Could you check a few things on this model? Use its own coordinates, in mm. Face numbers are marked on the shaded views. A direction names the side the tool comes from. Give positions to 0.01 mm unless a question says otherwise; leave off trailing zeros. Order: outer loops, then holes, each group sorted by start corner. A loop starts at its lowest first (then second) coordinate and runs counter-clockwise, first axis right, second up.
(1) If we mould it in two halves opening along Z, with no side actions, what happens to the marked faces 1, 2 and 3? For each: released by +Z, released by -Z, zero draft, split by the parting line, or undercut.
(2) Imagine slicing it at B-B, the plane z = 4.75. Write out the boundary of the cut face in (x, y).
(3) Imagine slicing it at C-C, the plane x = 11. Write out the boundary of the cut face in (y, z).
(4) If I drill on probe 1 along X at (y, z) = (3, -1); probe 2 along Z at (x, y) = (-15, 3); probe 3 along Z at (x, y) = (19, 5.75), over which ranges is the centre line in solid material (lowest first)?
(5) Imagine slicing it at A-A, the plane y = 4.5. Write out the boundary of the cut face in (x, z), then the cut area to 3 significant figures.
(6) Imagine slicing it at D-D, the plane z = 2. Write out the boundary of the cut face in (x, y), then the cut area to 3 significant figures.
(7) Will these pins go through, and if not, where does the flat tip stop? pin 1 (1 mm diameter, centred on y = 4.5, z = -7, fed in from +X); pin 2 (11 mm diameter, centred on x = 10.5, z = -1.5, fed in from +Y); pin 3 (1.6 mm diameter, centred on y = 4.5, z = -8, fed in from -X).
(8) On a 3-axis mill with a long thin cutter (end or side, diameter ignored), from which of +Z, -Z, +X, -X, +Y, -Y can I reach the whole of each face in a straight line? I mean the marked faces 4 and 5. Say none if no direction works.
from build123d import *

# Parameters (mm, degrees)
SKETCH_1_W          = 42
SKETCH_1_H          = 25
EXTRUDE_1_DEPTH     = 3.1
SKETCH_3_R          = 1.15
CUT_EXTRUDE_1_DEPTH = 33.796493715
SKETCH_5_W          = 15.7
SKETCH_5_H          = 8.3
CUT_EXTRUDE_3_DEPTH = 1.6
FILLET_4_R          = 3
SKETCH_10_W         = 1.324084548
SKETCH_10_H         = 8.3
CUT_EXTRUDE_4_DEPTH = 0.7
CUT_EXTRUDE_5_DEPTH = 1.6
FILLET_5_R          = 0.3
CHAMFER_1_SIZE      = 0.4
CHAMFER_2_SIZE      = 2
FILLET_6_R          = 2
SKETCH_13_W         = 1
SKETCH_13_H         = 3.2
EXTRUDE_2_DEPTH     = 4.95
EXTRUDE_3_DEPTH     = 3.2
FILLET_7_R          = 0.2
FILLET_8_R          = 0.2


with BuildPart() as part:
    # 草图1 → 凸台-拉伸1 (new body)
    with BuildSketch(Plane(origin=(0, 0, 0), x_dir=(1, 0, 0), z_dir=(0, 1, 0))):
        Rectangle(SKETCH_1_W, SKETCH_1_H)
    extrude(amount=EXTRUDE_1_DEPTH)

    # 草图3 → 切除-拉伸1 (cut, through all)
    with BuildSketch(Plane.XY.offset(12.5)):
        with Locations((-5.97, 3.1)):
            Circle(SKETCH_3_R)
    extrude(amount=-CUT_EXTRUDE_1_DEPTH, mode=Mode.SUBTRACT)

    # 草图5 → 切除-拉伸3 (cut)
    with BuildSketch(Plane(origin=(0, 3.1, 0), x_dir=(1, 0, 0), z_dir=(0, 1, 0))):
        with Locations((3.58, 0.65)):
            Rectangle(SKETCH_5_W, SKETCH_5_H)
    extrude(amount=-CUT_EXTRUDE_3_DEPTH, mode=Mode.SUBTRACT)

    # 圆角4
    fillet_4_edges = [part.edges().sort_by_distance(p)[0] for p in [
        (-21, 1.55, 12.5),
        (21, 1.55, 12.5),
    ]]
    fillet(fillet_4_edges, radius=FILLET_4_R)

    # 草图10 → 切除-拉伸4 (cut)
    with BuildSketch(Plane(origin=(0, 3.1, 0), x_dir=(1, 0, 0), z_dir=(0, 1, 0))):
        with Locations((-4.932042274, 0.65)):
            Rectangle(SKETCH_10_W, SKETCH_10_H)
    extrude(amount=-CUT_EXTRUDE_4_DEPTH, mode=Mode.SUBTRACT)

    # 草图11 → 切除-拉伸5 (cut)
    with BuildSketch(Plane(origin=(0, 3.1, 0), x_dir=(1, 0, 0), z_dir=(0, 1, 0))):
        with BuildLine():
            Line((-3.32, -11), (-3.32, 11))
            Line((-3.32, 11), (19.5, 11))
            Line((19.5, 11), (19.5, -9.5))
            ThreePointArc((19.5, -9.5), (19.060660172, -10.560660172), (18, -11))
            Line((18, -11), (-3.32, -11))
        make_face()
        with BuildLine():
            Line((-19.5, 11), (-8.62, 11))
            Line((-8.62, 11), (-8.62, -11))
            Line((-8.62, -11), (-18, -11))
            ThreePointArc((-18, -11), (-19.060660172, -10.560660172), (-19.5, -9.5))
            Line((-19.5, -9.5), (-19.5, 11))
        make_face()
    extrude(amount=-CUT_EXTRUDE_5_DEPTH, mode=Mode.SUBTRACT)

    # 圆角5
    fillet_5_edges = [part.edges().sort_by_distance(p)[0] for p in [
        (-5.97, 1.95, 12.5),
    ]]
    fillet(fillet_5_edges, radius=FILLET_5_R)

    # 倒角1
    chamfer_1_edges = [part.edges().sort_by_distance(p)[0] for p in [
        (-4.881015028, 2.730389757, 3.5),
        (-4.881015028, 2.730389757, -4.8),
    ]]
    chamfer(chamfer_1_edges, length=CHAMFER_1_SIZE)

    # 倒角2
    # the kernel refuses this chamfer: 2 mm, written as the material it takes off along each edge
    with BuildSketch(Plane(origin=(-5.97, 3.1, -12.5), x_dir=(-0.0031415874858793974, 0.9999950652018581, 0), z_dir=(0.9999950652018581, 0.0031415874858793974, 0))) as chamfer_2_piece_1:
        Polygon((1.15, CHAMFER_2_SIZE), (1.15 + CHAMFER_2_SIZE, 0), (1.15, 0), align=None)
    revolve(axis=Axis((-5.97, 3.1, -12.5), (0, 0, 1)), revolution_arc=359.64, mode=Mode.SUBTRACT)

    # 圆角6
    fillet_6_edges = [part.edges().sort_by_distance(p)[0] for p in [
        (-3.32, 2.3, -11),
        (-8.62, 2.3, -11),
    ]]
    fillet(fillet_6_edges, radius=FILLET_6_R)

    # 草图13 → 凸台-拉伸2 (add)
    with BuildSketch(Plane.XZ.offset(-1.5)):
        with Locations((19, 7.85)):
            Rectangle(SKETCH_13_W, SKETCH_13_H)
        with Locations((19, -7.85)):
            Rectangle(SKETCH_13_W, SKETCH_13_H)
        with Locations((-19, -7.85)):
            Rectangle(SKETCH_13_W, SKETCH_13_H)
        with Locations((-19, 7.85)):
            Rectangle(SKETCH_13_W, SKETCH_13_H)
    extrude(amount=-EXTRUDE_2_DEPTH)

    # 草图14 → 凸台-拉伸3 (add)
    with BuildSketch(Plane(origin=(0, 0, -9.45), x_dir=(-1, 0, 0), z_dir=(0, 0, -1))):
        Polygon((-19.5, 6.45), (-19.5, 5.15), (-20.1, 5.15), (-20.1, 5.65), align=None)
        Polygon((20.1, 5.65), (19.5, 6.45), (19.5, 5.15), (20.1, 5.15), align=None)
    extrude_3 = extrude(amount=-EXTRUDE_3_DEPTH)

    # 镜向1: 凸台-拉伸3 across plane
    add(extrude_3.mirror(Plane.XY))

    # 圆角7
    fillet_7_edges = [part.edges().sort_by_distance(p)[0] for p in [
        (-21, 1.55, -12.5),
        (21, 1.55, -12.5),
    ]]
    fillet(fillet_7_edges, radius=FILLET_7_R)

    # 圆角8
    # the kernel refuses this fillet: 0.2 mm, written as the material it takes off along each edge
    with BuildSketch(Plane(origin=(-20.8, 0, -12.3), x_dir=(0, 0, -1), z_dir=(1, 0, 0))) as fillet_8_piece_1:
        with BuildLine():
            CenterArc((0.2 - FILLET_8_R, FILLET_8_R), FILLET_8_R, 270, 90)
            Line((0.2, FILLET_8_R), (0.2 + FILLET_8_R * 0.02, FILLET_8_R))
            Line((0.2 + FILLET_8_R * 0.02, FILLET_8_R), (0.2 + FILLET_8_R * 0.02, -FILLET_8_R * 0.02))
            Line((0.2 + FILLET_8_R * 0.02, -FILLET_8_R * 0.02), (0.2 - FILLET_8_R, -FILLET_8_R * 0.02))
            Line((0.2 - FILLET_8_R, -FILLET_8_R * 0.02), (0.2 - FILLET_8_R, 0))
        make_face()
    revolve(axis=Axis((-20.8, 0, -12.3), (0, 1, 0)), revolution_arc=90, mode=Mode.SUBTRACT)
    with BuildSketch(Plane(origin=(-21, 0, 9.5), x_dir=(1, 0, 0), z_dir=(0, 0, -1))) as fillet_8_piece_2:
        with BuildLine():
            CenterArc((FILLET_8_R, -FILLET_8_R), FILLET_8_R, 90, 90)
            Line((0, -FILLET_8_R), (-FILLET_8_R * 0.02, -FILLET_8_R))
            Line((-FILLET_8_R * 0.02, -FILLET_8_R), (-FILLET_8_R * 0.02, FILLET_8_R * 0.02))
            Line((-FILLET_8_R * 0.02, FILLET_8_R * 0.02), (FILLET_8_R, FILLET_8_R * 0.02))
            Line((FILLET_8_R, FILLET_8_R * 0.02), (FILLET_8_R, 0))
        make_face()
    extrude(amount=21.8, mode=Mode.SUBTRACT)
    with BuildSketch(Plane(origin=(-18, 0, 9.5), x_dir=(-1, 0, 0), z_dir=(0, 0, -1))) as fillet_8_piece_3:
        with BuildLine():
            CenterArc((3 - FILLET_8_R, FILLET_8_R), FILLET_8_R, 270, 90)
            Line((3, FILLET_8_R), (3 + FILLET_8_R * 0.02, FILLET_8_R))
            Line((3 + FILLET_8_R * 0.02, FILLET_8_R), (3 + FILLET_8_R * 0.02, -FILLET_8_R * 0.02))
            Line((3 + FILLET_8_R * 0.02, -FILLET_8_R * 0.02), (3 - FILLET_8_R, -FILLET_8_R * 0.02))
            Line((3 - FILLET_8_R, -FILLET_8_R * 0.02), (3 - FILLET_8_R, 0))
        make_face()
    revolve(axis=Axis((-18, 0, 9.5), (0, 1, 0)), revolution_arc=90, mode=Mode.SUBTRACT)
    with BuildSketch(Plane(origin=(18, 0, 12.5), x_dir=(0, 1, 0), z_dir=(-1, 0, 0))) as fillet_8_piece_4:
        with BuildLine():
            CenterArc((FILLET_8_R, FILLET_8_R), FILLET_8_R, 180, 90)
            Line((0, FILLET_8_R), (-FILLET_8_R * 0.02, FILLET_8_R))
            Line((-FILLET_8_R * 0.02, FILLET_8_R), (-FILLET_8_R * 0.02, -FILLET_8_R * 0.02))
            Line((-FILLET_8_R * 0.02, -FILLET_8_R * 0.02), (FILLET_8_R, -FILLET_8_R * 0.02))
            Line((FILLET_8_R, -FILLET_8_R * 0.02), (FILLET_8_R, 0))
        make_face()
    extrude(amount=36, mode=Mode.SUBTRACT)
    with BuildSketch(Plane(origin=(18, 0, 9.5), x_dir=(0, 0, 1), z_dir=(-1, 0, 0))) as fillet_8_piece_5:
        with BuildLine():
            CenterArc((3 - FILLET_8_R, FILLET_8_R), FILLET_8_R, 270, 90)
            Line((3 - FILLET_8_R, 0), (3 - FILLET_8_R, -FILLET_8_R * 0.02))
            Line((3 - FILLET_8_R, -FILLET_8_R * 0.02), (3 + FILLET_8_R * 0.02, -FILLET_8_R * 0.02))
            Line((3 + FILLET_8_R * 0.02, -FILLET_8_R * 0.02), (3 + FILLET_8_R * 0.02, FILLET_8_R))
            Line((3 + FILLET_8_R * 0.02, FILLET_8_R), (3, FILLET_8_R))
        make_face()
    revolve(axis=Axis((18, 0, 9.5), (0, 1, 0)), revolution_arc=90, mode=Mode.SUBTRACT)
    with BuildSketch(Plane(origin=(21, 0, -12.3), x_dir=(0, 1, 0), z_dir=(0, 0, 1))) as fillet_8_piece_6:
        with BuildLine():
            CenterArc((FILLET_8_R, FILLET_8_R), FILLET_8_R, 180, 90)
            Line((0, FILLET_8_R), (-FILLET_8_R * 0.02, FILLET_8_R))
            Line((-FILLET_8_R * 0.02, FILLET_8_R), (-FILLET_8_R * 0.02, -FILLET_8_R * 0.02))
            Line((-FILLET_8_R * 0.02, -FILLET_8_R * 0.02), (FILLET_8_R, -FILLET_8_R * 0.02))
            Line((FILLET_8_R, -FILLET_8_R * 0.02), (FILLET_8_R, 0))
        make_face()
    extrude(amount=21.8, mode=Mode.SUBTRACT)
    with BuildSketch(Plane(origin=(20.8, 0, -12.3), x_dir=(0, 0, -1), z_dir=(-1, 0, 0))) as fillet_8_piece_7:
        with BuildLine():
            CenterArc((0.2 - FILLET_8_R, -FILLET_8_R), FILLET_8_R, 0, 90)
            Line((0.2 - FILLET_8_R, 0), (0.2 - FILLET_8_R, FILLET_8_R * 0.02))
            Line((0.2 - FILLET_8_R, FILLET_8_R * 0.02), (0.2 + FILLET_8_R * 0.02, FILLET_8_R * 0.02))
            Line((0.2 + FILLET_8_R * 0.02, FILLET_8_R * 0.02), (0.2 + FILLET_8_R * 0.02, -FILLET_8_R))
            Line((0.2 + FILLET_8_R * 0.02, -FILLET_8_R), (0.2, -FILLET_8_R))
        make_face()
    revolve(axis=Axis((20.8, 0, -12.3), (0, -1, 0)), revolution_arc=90, mode=Mode.SUBTRACT)
    with BuildSketch(Plane(origin=(-6.610983006, 0, -12.5), x_dir=(0, 1, 0), z_dir=(1, 0, 0))) as fillet_8_piece_8:
        with BuildLine():
            CenterArc((FILLET_8_R, FILLET_8_R), FILLET_8_R, 180, 90)
            Line((0, FILLET_8_R), (-FILLET_8_R * 0.02, FILLET_8_R))
            Line((-FILLET_8_R * 0.02, FILLET_8_R), (-FILLET_8_R * 0.02, -FILLET_8_R * 0.02))
            Line((-FILLET_8_R * 0.02, -FILLET_8_R * 0.02), (FILLET_8_R, -FILLET_8_R * 0.02))
            Line((FILLET_8_R, -FILLET_8_R * 0.02), (FILLET_8_R, 0))
        make_face()
    extrude(amount=27.410983006, mode=Mode.SUBTRACT)
    with BuildSketch(Plane(origin=(-20.8, 0, -12.5), x_dir=(0, 0, 1), z_dir=(1, 0, 0))) as fillet_8_piece_9:
        with BuildLine():
            CenterArc((FILLET_8_R, -FILLET_8_R), FILLET_8_R, 90, 90)
            Line((0, -FILLET_8_R), (-FILLET_8_R * 0.02, -FILLET_8_R))
            Line((-FILLET_8_R * 0.02, -FILLET_8_R), (-FILLET_8_R * 0.02, FILLET_8_R * 0.02))
            Line((-FILLET_8_R * 0.02, FILLET_8_R * 0.02), (FILLET_8_R, FILLET_8_R * 0.02))
            Line((FILLET_8_R, FILLET_8_R * 0.02), (FILLET_8_R, 0))
        make_face()
    extrude(amount=15.470983006, mode=Mode.SUBTRACT)


solid = part.part
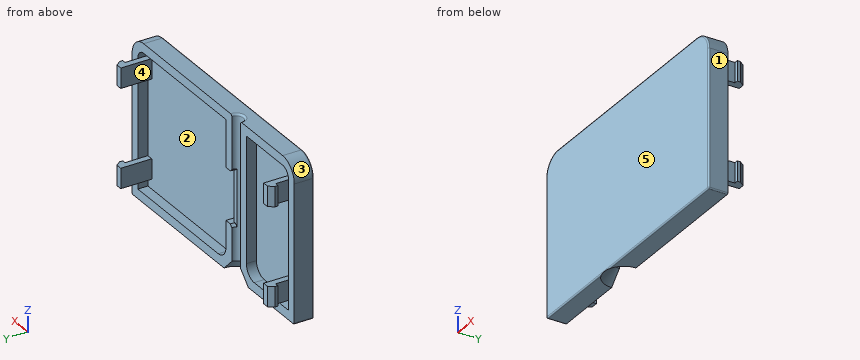
Answer block:
1. face 1: zero draft
1. face 2: undercut
1. face 3: released by +Z
2. outline: (-21, 0.2) arc R0.2 ccw to (-20.8, 0) - (20.8, 0) arc R0.2 ccw to (21, 0.2) - (21, 3.1) - (19.5, 3.1) - (19.5, 1.5) - (-3.32, 1.5) - (-3.32, 3.1) - (-4.82, 3.1) arc R1.15 cw to (-7.12, 3.1) - (-8.62, 3.1) - (-8.62, 1.5) - (-19.5, 1.5) - (-19.5, 3.1) - (-21, 3.1) - close
3. outline: (0, -12.3) arc R0.2 ccw to (0.2, -12.5) - (3.1, -12.5) - (3.1, -11) - (1.5, -11) - (1.5, 11) - (3.1, 11) - (3.1, 12.5) - (0.2, 12.5) arc R0.2 ccw to (0, 12.3) - close
4. probe 1: x = -21 to -19.5, -8.62 to -7.12, 19.5 to 21
4. probe 2: z = -12.5 to -11, 11 to 12.5
4. probe 3: z = -9.45 to -6.25, 6.25 to 9.45
5. outline: (-19.5, -9.45) - (-18.5, -9.45) - (-18.5, -6.25) - (-19.5, -6.25) - close; (-19.5, 6.25) - (-18.5, 6.25) - (-18.5, 9.45) - (-19.5, 9.45) - close; (18.5, -9.45) - (19.5, -9.45) - (19.5, -6.25) - (18.5, -6.25) - close; (18.5, 6.25) - (19.5, 6.25) - (19.5, 9.45) - (18.5, 9.45) - close
5. area: 12.8 mm2
6. outline: (-21, 0.2) arc R0.2 ccw to (-20.8, 0) - (20.8, 0) arc R0.2 ccw to (21, 0.2) - (21, 3.1) - (19.5, 3.1) - (19.5, 1.5) - (-4.27, 1.5) - (-4.27, 2.4) - (-5.06, 2.4) arc R1.15 cw to (-7.12, 3.1) - (-8.62, 3.1) - (-8.62, 1.5) - (-19.5, 1.5) - (-19.5, 3.1) - (-21, 3.1) - close
6. area: 72.2 mm2
7. pin 1: stops at x = 19.5
7. pin 2: stops at y = 1.5
7. pin 3: stops at x = -20.1
8. face 4: +Y
8. face 5: +Z, -Z, +X, -X, -Y
